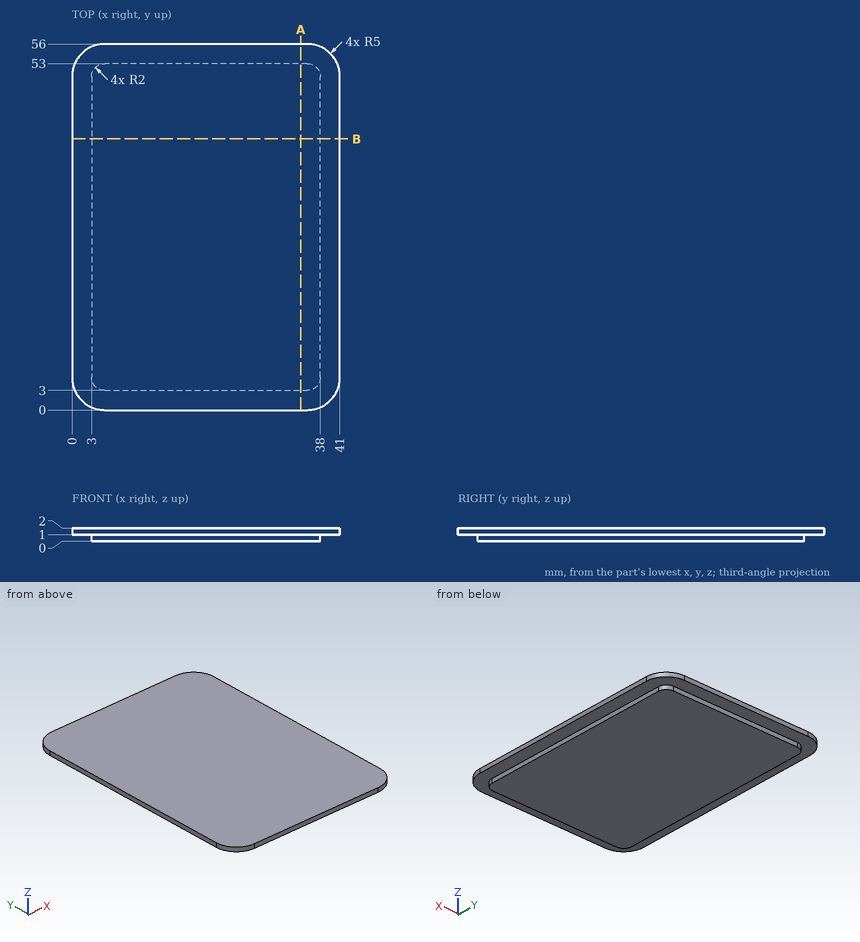
Design review of the part shown in the three views and the two pictorial views. Dimensions are in mm from the part's minimum x, y and z. Coordinates: 2 decimals unless noted, no trailing zeros. Write each loop counter-clockwise with the first axis right and the second up, starting at its lowest first coordinate (ties: lowest second). Pieces come first, ordered by that corner, then holes.
1) We need section B-B on y = 41.5. State the section outline as (x, z) points, then the cut area to 3 significant figures.
2) Clearance check with flat-ended pins moving along their axes: pin 1 Ø0.8 at (x, z) = (21.5, 0.5) entering from -Y; pin 2 Ø0.8 at (y, z) = (26, 0.5) entering from -X. State where each tip first meets the part, or that it passes through.
3) We need section A-A on x = 35. State the section outline as (y, z) points.
4) To check wall thickness, follow probe 1 along Y at (x, z) = (23, 0.8); probe 2 along X at (y, z) = (24, 0.85); probe 3 along Z at (x, y) = (2, 28). State the ranges of each line that lie inside material, in increasing order.
Answer list:
1. outline: (0, 1) - (3, 1) - (3, 0) - (38, 0) - (38, 1) - (41, 1) - (41, 2) - (0, 2) - close
1. area: 76.0 mm2
2. pin 1: stops at y = 3
2. pin 2: stops at x = 3
3. outline: (0, 1) - (3, 1) - (3, 0) - (53, 0) - (53, 1) - (56, 1) - (56, 2) - (0, 2) - close
4. probe 1: y = 3 to 53
4. probe 2: x = 3 to 38
4. probe 3: z = 1 to 2
